from build123d import *

# Parameters (mm, degrees)
ESQUISSE1_W             = 130
ESQUISSE1_H             = 40
BOSS_EXTRU_1_DEPTH      = 6
ESQUISSE5_W             = 50
ESQUISSE5_H             = 6
BOSS_EXTRU_3_DEPTH      = 6
ENL_V_MAT_EXTRU_1_DEPTH = 47


with BuildPart() as part:
    # Esquisse1 → Boss.-Extru.1 (new body)
    with BuildSketch(Plane.XY):
        Rectangle(ESQUISSE1_W, ESQUISSE1_H)
    extrude(amount=BOSS_EXTRU_1_DEPTH)

    # Esquisse5 → Boss.-Extru.3 (add)
    with BuildSketch(Plane(origin=(0, 0, 0), x_dir=(-1, 0, 0), z_dir=(0, 0, -1))):
        with Locations((0, 23)):
            Rectangle(ESQUISSE5_W, ESQUISSE5_H)
        with Locations((0, -23)):
            Rectangle(ESQUISSE5_W, ESQUISSE5_H)
    extrude(amount=-BOSS_EXTRU_3_DEPTH)

    # Esquisse6 → Enlèv. mat.-Extru.1 (cut, through all)
    with BuildSketch(Plane.XZ.offset(20)):
        Polygon((65, 6), (45, 0), (65, 0), align=None)
    extrude(amount=-ENL_V_MAT_EXTRU_1_DEPTH, mode=Mode.SUBTRACT)


solid = part.part
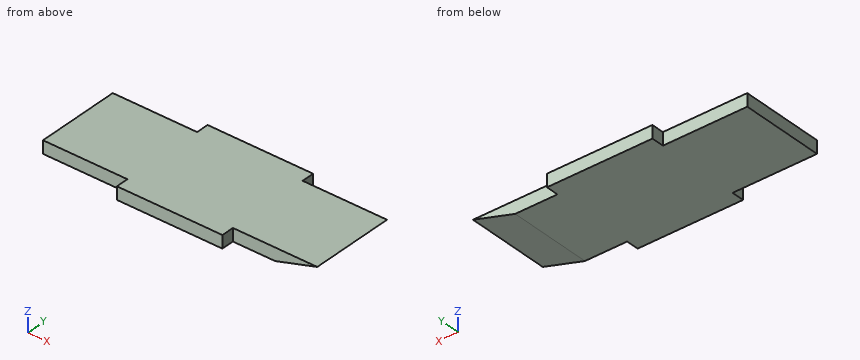
Verification items for the finished model (mm, model axes). Coordinates: 2 decimals unless noted, no trailing zeros. Order: outer loops, then holes, each group sorted by start corner. A loop starts at its lowest first (then second) coordinate and runs counter-clockwise, first axis right, second up. Notation, with made-up numbers: M 16.25,17.25 L 49.25,17.25 A20 cw 49.25,53.25 Z; hole C -33.5,-8 d6. An arc over 180 degrees is marked long. Write each question's results on one line, items separated by ' | '.
1) Section check A-A on z = 1.5. Record the cut outline in (x, y).
Solved:
outline: M -65,-20 L -25,-20 L -25,-26 L 25,-26 L 25,-20 L 50,-20 L 50,20 L 25,20 L 25,26 L -25,26 L -25,20 L -65,20 Z
2) Section check C-C on y = 6.5. Record the cut outline in (x, z).
Solved:
outline: M -65,0 L 45,0 L 65,6 L -65,6 Z
3) Scan lines: line 1 along Y through (x, z) = (26.5, 0.75); line 2 along X through (y, z) = (23, 3.5). Record each from-to range of solid material in increasing order. Write a range as [from, to].
Solved:
line 1: y = [-20, 20] | line 2: x = [-25, 25]
4) Gauge pin test, flat ends, axial feed: pin 1 Ø3 at (x, z) = (46, 2) entering from +Y; pin 2 Ø3 at (x, z) = (-39.5, 3.5) entering from -Y; pin 3 Ø1.8 at (y, z) = (-24, 2) entering from -X. Record the tip position at first contact, or that the pin passes through.
Solved:
pin 1: stops at y = 20 | pin 2: stops at y = -20 | pin 3: stops at x = -25
5) Section check B-B on x = 49. Record the cut outline in (y, z), plus the area to 3 significant figures.
Solved:
outline: M -20,1.2 L 20,1.2 L 20,6 L -20,6 Z | area: 192 mm²
